Model file for the job. Use its own axes, mm. A direction names the side the tool comes from. Give positions to 0.01 mm unless a question says otherwise; leave off trailing zeros. Answer in a Markdown table with one row per item.
Autodesk Inventor part; units mm, degrees
sketch "Эскиз2" plane through (0, 0, 0) normal (0, 1, 0) x (-1, 0, 0)
  line L0 (105, 150) -> (-105, 150)
  line L1 (-105, 150) -> (-105, -150)
  line L2 (-105, -150) -> (105, -150)
  line L3 (105, -150) -> (105, 150)
  line L4 (105, 150) -> (-105, -150) construction
  line L5 (-105, 150) -> (105, -150) construction
  point P0 (0, 0)
  dimension "d0" = 300
  dimension "d1" = 210
extrude "Выдавливание1" add sketch "Эскиз2" along normal mid plane 4
sketch "Эскиз4" plane through (0, 2, 0) normal (0, 1, 0) x (1, 0, 0)
  point P0 (0, 0)
sketch "Эскиз5" plane through (0, -2, 0) normal (0, -1, 0) x (1, 0, 0)
  line L0 (46.7, -140) -> (-46.7, -140)
  line L1 (-46.7, -140) -> (-46.7, -121.5234)
  arc A0 (-46.594, -118.6405) -> (-46.7, -121.5234) centre (-7.4334, -121.5237) ccw
  ellipse E0 centre (-51.6674, -118.2652) end of major axis (-52.1006, -124.2245) minor radius 5.0873 (-46.594, -118.6405) -> (-46.5935, -117.6187) ccw
  ellipse E1 centre (-32.0119, -116.0476) end of major axis (-31.7353, -98.7858) minor radius 14.6347 (-46.6171, -115.0294) -> (-46.5935, -117.6187) ccw
  spline S0 degree 3 poles (-46.6171, -115.0294) (-46.5015, -112.9122) (-46.0285, -108.6931) (-44.8405, -103.5371) (-43.2174, -98.5282) (-41.5773, -94.6618) (-39.1217, -90.0608) (-36.8431, -86.5874) (-33.6324, -82.5567) (-30.7879, -79.6008) (-26.9267, -76.2879) (-23.6107, -73.9602) (-19.2299, -71.4921) (-15.5575, -69.8842) (-10.8129, -68.3603) (-6.9178, -67.5387) (-1.9855, -67.0233) (1.9855, -67.0233) (6.9178, -67.5387) (10.8129, -68.3603) (15.5575, -69.8842) (19.2299, -71.4921) (23.6107, -73.9602) (26.9267, -76.2879) (30.7879, -79.6008) (33.6324, -82.5567) (36.8431, -86.5874) (39.1217, -90.0608) (41.5773, -94.6618) (43.2174, -98.5282) (44.8405, -103.5371) (46.0285, -108.6931) (46.5015, -112.9122) (46.6171, -115.0294) knots 1.630961 1.630961 1.630961 1.630961 1.756847 1.882733 1.945676 2.071562 2.134505 2.260391 2.323334 2.44922 2.512163 2.638049 2.700992 2.826878 2.889821 3.015707 3.07865 3.204536 3.267479 3.393365 3.456308 3.582194 3.645137 3.771023 3.833966 3.959852 4.022795 4.148681 4.211624 4.33751 4.400453 4.526339 4.652225 4.652225 4.652225 4.652225
  ellipse E2 centre (32.0119, -116.0476) end of major axis (31.7353, -98.7858) minor radius 14.6347 (46.5935, -117.6187) -> (46.6171, -115.0294) ccw
  ellipse E3 centre (51.6674, -118.2652) end of major axis (52.1006, -124.2245) minor radius 5.0873 (46.5935, -117.6187) -> (46.594, -118.6405) ccw
  arc A1 (46.7, -121.5234) -> (46.594, -118.6405) centre (7.4334, -121.5237) ccw
  line L2 (46.7, -121.5234) -> (46.7, -140)
  line L3 (38.7, -118.0685) -> (38.7, -133.5234)
  ellipse E4 centre (0, -118.0685) end of major axis (0, -75.3678) minor radius 38.7 (38.7, -118.0685) -> (-38.7, -118.0685) ccw
  line L4 (-38.7, -133.5234) -> (-38.7, -118.0685)
  line L5 (-21.135, -133.5234) -> (-38.7, -133.5234)
  circle A2 centre (9.4549, -127.5234) radius 2.1
  circle A3 centre (0, -118.0685) radius 2.1
  circle A4 centre (-9.4549, -127.5234) radius 2.1
  circle A5 centre (9.4549, -127.5234) radius 1.5
  circle A6 centre (-9.4549, -127.5234) radius 1.5
  circle A7 centre (0, -118.0685) radius 1.5
  line L6 (39.7, -118.0685) -> (39.7, -134.4459)
  line L7 (-39.7, -133.5234) -> (-39.7, -118.0685)
  line L8 (38.7, -133.5234) -> (39.7, -133.5234)
  line L9 (-38.7, -133.5234) -> (-39.7, -133.5234)
  line L10 (38.7, -133.5234) -> (21.135, -133.5234)
  line L11 (9.7861, -111.8345) -> (21.135, -133.5234)
  ellipse E5 centre (0, -118.0685) end of major axis (0, -105.6004) minor radius 11.3 (9.7861, -111.8345) -> (-9.7861, -111.8345) ccw
  line L12 (-21.135, -133.5234) -> (-9.7861, -111.8345)
  spline S1 degree 5 poles (-39.7, -118.0685) (-39.7, -116.2442) (-39.6135, -114.4198) (-39.4406, -112.6008) (-38.359, -105.0548) (-35.7799, -97.7978) (-32.9708, -92.6223) (-25.8915, -83.6065) (-16.2115, -77.5088) (-10.9886, -75.4127) (0, -73.3231) (10.9886, -75.4127) (16.2115, -77.5088) (25.8915, -83.6065) (32.9708, -92.6223) (35.7799, -97.7978) (38.359, -105.0548) (39.4406, -112.6008) (39.6135, -114.4198) (39.7, -116.2442) (39.7, -118.0685) knots 0 0 0 0 0 0 0.069589 0.069589 0.069589 0.290442 0.290442 0.290442 0.5 0.5 0.5 0.709558 0.709558 0.709558 0.930411 0.930411 0.930411 1 1 1 1 1 1
  point P0 (0, 0)
  dimension "d18" = 1
  dimension "d15" = 3
  dimension "d16" = 3
  dimension "d17" = 3
extrude "Выдавливание3" cut sketch "Эскиз5" against normal blind 10 contours E4 L4 L9 L7 S1 L6 L8 L3 | L3 L10 L11 E5 L12 L5 L4 E4 | A5 | A6 | A7
sketch "Эскиз6" plane through (0, -2, 0) normal (0, -1, 0) x (1, 0, 0)
  circle A0 centre (95, -110) radius 2.5
  circle A1 centre (95, -40) radius 2.5
  circle A2 centre (95, 25) radius 2.5
  circle A3 centre (95, 75) radius 2.5
  circle A4 centre (95, 125) radius 2.5
  circle A5 centre (-95, -110) radius 2.5
  circle A6 centre (-95, -40) radius 2.5
  circle A7 centre (-95, 25) radius 2.5
  circle A8 centre (-95, 75) radius 2.5
  circle A9 centre (-95, 125) radius 2.5
  point P0 (0, 0)
extrude "Выдавливание4" cut sketch "Эскиз6" against normal up to next
properties part number "Передняя_фанера"
(1) Saw through at A-A, the plane y = -1.1. Count the separate pieces of the cut face and the enclosed holes in it, and give its area (3 significant figures).
Established:
| item | result |
|---|---|
| separate pieces | 1 |
| enclosed holes | 14 |
| area | 59,600 mm2 |
(2) Wall check: L1, parallel to Z at x = 95, y = -0.7; L2, parallel to Z at x = 0, y = 0.9; L3, parallel to X at y = -1.8, z = -117.5. Give the ranges that are in metal, low to high.
Established:
| item | result |
|---|---|
| L1 | z = -150 to -112.5, -107.5 to -42.5, -37.5 to 22.5, 27.5 to 72.5, 77.5 to 122.5, 127.5 to 150 |
| L2 | z = -150 to -119.57, -116.57 to -105.6, -74.37 to 150 |
| L3 | x = -105 to -39.7, -12.75 to -1.39, 1.39 to 12.75, 39.7 to 105 |
(3) Which spindle directions (+Z, -Z, +X, -X, +Y, -Y) get a long thin tool onto all of the face, cutting with end or side? Do faces 1 (the flat face through (1, -2, 2)), 2 (the flat face through (-15.54, -0.03, -122.83)). Say none if no direction does.
Established:
| item | result |
|---|---|
| face 1 | +Z, -Z, +X, -X, -Y |
| face 2 | +Y, -Y |
